Here's how the part is built. I have some questions about the finished solid (model axes, mm). A direction names the side the tool comes from. Round coordinates to 2 decimals unless told otherwise and drop trailing zeros. Put each result on its own line as item: value. Start each with the question number.
1. I need wall thicknesses on probe 1 along X at (y, z) = (-58.4, 8); probe 2 along Y at (x, z) = (-12, 14); probe 3 along Y at (x, z) = (-8, 32). Which ranges of each line are inside material? Lowest first, please. Write a range as from..to.
2. For pin 1 (3 mm diameter, centred on x = 2.5, z = 22, fed in from +Y); pin 2 (3 mm diameter, centred on x = -11.05, z = 55, fed in from -Y); pin 3 (5.5 mm diameter, centred on y = 18, z = 34, fed in from +X), each with a flat end and sliding along its axis, tell me the tip position at first contact or that it passes through.
3. Which directions (+Z, -Z, +X, -X, +Y, -Y) give clear straight access to the entire face, cutting with the end or side of a thin tool? Please do faces 4 (the face through (-15.046, -58, 31)), 5 (the face through (-10, -55.81, 32)), 6 (the face through (-8.046, 19, 3)).
4. Suppose I cut it at A-A (z = 8). Count the separate pieces of the cut face and the enclosed holes in it, then the cut area to 3 significant figures.
5. We'd pull the mould along Y, two halves only. Please class faces 1 (the face through (-16.856, -16.116, 31.059)), 2 (the face through (-8.046, 19, 60)), 3 (the face through (-22.44, -0.866, 31.059)): +Y half, -Y half, draft (parallel to the pull), parting line (faces both ways), or undercut.
```python
from build123d import *

# Parameters (mm, degrees)
BOSS_EXTRUDE1_DEPTH = 63
SKETCH12_W          = 10
SKETCH12_H          = 63
BOSS_EXTRUDE6_DEPTH = 5
BOSS_EXTRUDE7_DEPTH = 63
FILLET4_R           = 5
SKETCH14_R          = 2
CUT_EXTRUDE5_DEPTH  = 10
SKETCH15_R          = 4
SKETCH15_R_2        = 2
BOSS_EXTRUDE8_DEPTH = 5
SKETCH16_W          = 20
SKETCH16_H          = 63
BOSS_EXTRUDE9_DEPTH = 5
FILLET5_R           = 5
CUT_EXTRUDE6_START  = -5
SKETCH17_R          = 2
CUT_EXTRUDE6_DEPTH  = 5
CUT_EXTRUDE7_DEPTH  = 80
FILLET6_R           = 10


# Read off the part's stored shape, not the designer's step: Boss-Extrude1
with BuildPart() as part:
    # Boss-Extrude1 outline → Boss-Extrude1 (new body)
    with BuildSketch(Plane.XY):
        with BuildLine():
            Line((4.954113003, -60.810475982), (9.954113003, -60.810475982))
            add(Edge.make_bspline(
                [(9.954113003, -60.810475982), (1.787820041, -34.566500255), (-27.991304854, -7.282060069), (-18.045886997, 21.189524018)],
                knots=[0, 0, 0, 0, 1, 1, 1, 1], degree=3))
            Line((-18.045886997, 21.189524018), (-23.045886997, 21.189524018))
            add(Edge.make_bspline(
                [(-23.045886997, 21.189524018), (-23.192896954, 20.707388184), (-23.619107908, 19.21203202), (-24.398456673, 15.722733579), (-24.92594246, 10.71547172), (-24.705924446, 4.806399572), (-23.443795498, -2.907918287), (-20.364970108, -12.213873941), (-15.162719206, -22.926775882), (-9.22446855, -33.283941227), (-4.27318175, -41.652306471), (-0.670405229, -48.178299158), (1.765142475, -52.980809676), (3.499618766, -56.88928979), (4.492016037, -59.486726266), (4.856824136, -60.525956387), (4.954113003, -60.810475982)],
                knots=[0.016302379, 0.016302379, 0.016302379, 0.016302379, 0.03125, 0.0625, 0.125, 0.1875, 0.25, 0.375, 0.5, 0.625, 0.75, 0.8125, 0.875, 0.9375, 0.96875, 0.980543141, 0.980543141, 0.980543141, 0.980543141], degree=3))
        make_face()
    extrude(amount=BOSS_EXTRUDE1_DEPTH)



with BuildPart() as body_2:
    # Sketch12 → Boss-Extrude6 (new body)
    with BuildSketch(Plane(origin=(0, 21.189524018, 0), x_dir=(1, 0, 0), z_dir=(0, 1, 0))):
        with Locations((-13.045886997, -31.5)):
            Rectangle(SKETCH12_W, SKETCH12_H)
    extrude(amount=-BOSS_EXTRUDE6_DEPTH)


with BuildPart() as part_1:
    add(part.part)

    add(body_2.part)  # Boss-Extrude7 merges body 2
    # Sketch13 → Boss-Extrude7 (add)
    with BuildSketch(Plane.XY.offset(63)):
        with BuildLine():
            Line((-18.045886997, 16.189524018), (-18.045886997, 21.189524018))
            add(Edge.make_bspline(
                [(-19.398734896, 16.189524018), (-19.076313221, 17.852122544), (-18.629495341, 19.518779331), (-18.045886997, 21.189524018)],
                knots=[0.941318871, 0.941318871, 0.941318871, 0.941318871, 1, 1, 1, 1], degree=3))
            Line((-19.398734896, 16.189524018), (-18.045886997, 16.189524018))
        make_face()
    extrude(amount=-BOSS_EXTRUDE7_DEPTH)

    # Fillet4
    fillet4_edges = [part_1.edges().sort_by_distance(p)[0] for p in [
        (-19.398734896, 16.189524018, 31.5),
    ]]
    fillet(fillet4_edges, radius=FILLET4_R)

    # Sketch14 → Cut-Extrude5 (cut)
    with BuildSketch(Plane.XZ.offset(-16.189524018)):
        with Locations((-11.045886997, 8)):
            Circle(SKETCH14_R)
        with Locations((-11.045886997, 55)):
            Circle(SKETCH14_R)
    extrude(amount=-CUT_EXTRUDE5_DEPTH, mode=Mode.SUBTRACT)

    # Sketch15 → Boss-Extrude8 (add)
    # profile 1 of 2: a face of its own
    with BuildSketch(Plane.XZ.offset(-16.189524018)):
        with Locations((-11.045886997, 55)):
            Circle(SKETCH15_R)
        with Locations((-11.045886997, 55)):
            Circle(SKETCH15_R_2, mode=Mode.SUBTRACT)
    # profile 2 of 2: a face of its own
    with BuildSketch(Plane.XZ.offset(-16.189524018)):
        with Locations((-11.045886997, 8)):
            Circle(SKETCH15_R)
        with Locations((-11.045886997, 8)):
            Circle(SKETCH15_R_2, mode=Mode.SUBTRACT)
    extrude(amount=-BOSS_EXTRUDE8_DEPTH)

    # Sketch16 → Boss-Extrude9 (add)
    with BuildSketch(Plane.XZ.offset(60.810475982)):
        with Locations((-5.045886997, 31.5)):
            Rectangle(SKETCH16_W, SKETCH16_H)
    extrude(amount=-BOSS_EXTRUDE9_DEPTH)

    # Fillet5
    fillet5_edges = [part_1.edges().sort_by_distance(p)[0] for p in [
        (3.003762593, -55.810475982, 31.5),
    ]]
    fillet(fillet5_edges, radius=FILLET5_R)

    # Sketch17 → Cut-Extrude6 (cut)
    with BuildSketch(Plane(origin=(0, -55.810475982, 0), x_dir=(1, 0, 0), z_dir=(0, 1, 0)).offset(CUT_EXTRUDE6_START)):
        with Locations((-11.045886997, -55)):
            Circle(SKETCH17_R)
        with Locations((-11.045886997, -8)):
            Circle(SKETCH17_R)
    extrude(amount=CUT_EXTRUDE6_DEPTH, mode=Mode.SUBTRACT)

    # Sketch18 → Cut-Extrude7 (cut)
    with BuildSketch(Plane(origin=(0, 0, 0), x_dir=(-1, 0, 0), z_dir=(0, 0, -1))):
        Polygon((23.045886997, 1.542241973), (27.88763941, -1.261096589), (21.516415404, -20.247344126), (15.527464839, -18.463401404), align=None)
    extrude(amount=-CUT_EXTRUDE7_DEPTH, mode=Mode.SUBTRACT)

    # Fillet6
    # the kernel refuses this fillet: 10 mm, written as the material it adds along each edge
    with BuildSketch(Plane(origin=(-15.527464839, -18.463401404, 0), x_dir=(-0.958385683586268, -0.28547658660016567, 0), z_dir=(0, 0, 1))) as fillet6_piece_1:
        with BuildLine():
            CenterArc((10.361821719, -4.811763892), FILLET6_R, 151.237737935, 32.771900007)
            Line((0.386298698, -5.51100666), (0.186788237, -5.524991515))
            Line((0.186788237, -5.524991515), (-0.19951046, -0.013984855))
            Line((-0.19951046, -0.013984855), (0, 0.2))
            ThreePointArc((0, 0.2), (0.797791872, 0.2), (1.420258984, 0.096235278))
            Line((1.420258984, 0.096235278), (1.595583743, 0))
        make_face()
    extrude(amount=63)
    with BuildSketch(Plane(origin=(-23.045886997, 1.542241973, 0), x_dir=(0.35179225201059605, -0.9360781011354306, 0), z_dir=(0, 0, 1))) as fillet6_piece_2:
        with BuildLine():
            CenterArc((4.818055228, -10), FILLET6_R, 90, 27.571489076)
            Line((0.189505284, -1.1356599), (0.096934285, -0.958373098))
            ThreePointArc((0.096934285, -0.958373098), (-0.102519699, -0.600748389), (-0.197272341, -0.032918439))
            Line((-0.197272341, -0.032918439), (0, 0.2))
            Line((0, 0.2), (4.818055228, 0.2))
            Line((4.818055228, 0.2), (4.818055228, 0))
        make_face()
    extrude(amount=63)


solid = part_1.part
```
Verdict:
1. probe 1: x = -15.05..-13.05, -9.05..9.15
1. probe 2: y = -60.81..-55.81, -28.41..-18.4, 16.19..21.19
1. probe 3: y = -60.81..-55.81, -35.33..-25.82
2. pin 1: stops at y = -41.4
2. pin 2: stops at y = -32.67
2. pin 3: stops at x = -8.05
3. face 4: +Z, -Z, -X, -Y
3. face 5: +Z, -Z, -X
3. face 6: -Z, +X, +Y
4. separate pieces: 3
4. enclosed holes: 0
4. area: 522 mm^2
5. face 1: undercut
5. face 2: draft
5. face 3: -Y half
